Read the model definition and answer for the solid it produces. Units are mm, in the model's axes. A direction names the side the tool comes from. Coordinates: 2 decimals unless noted, no trailing zeros. Write each loop counter-clockwise with the first axis right and the second up, starting at its lowest first coordinate (ties: lowest second). Pieces come first, ordered by that corner, then holes. Notation, with made-up numbers: (2, -1) - (31, -1) arc R19 ccw to (31, 14) - close; hole circle Ø4 at (36, -5). An arc over 180 degrees is marked (long way). Use a Markdown table: item, result.
from build123d import *

# Parameters (mm, degrees)
SKETCH1_R           = 14.2875
SKETCH1_R_2         = 2.6289
BOSS_EXTRUDE1_DEPTH = 6.35


with BuildPart() as part:
    # Sketch1 → Boss-Extrude1 (new body)
    with BuildSketch(Plane(origin=(0, 0, 0), x_dir=(0, 0, -1), z_dir=(1, 0, 0))):
        with BuildLine():
            Line((-12.7, -12.7), (-88.9, -12.7))
            Line((-88.9, -12.7), (-122.826729432, 47.599537172))
            ThreePointArc((-122.826729432, 47.599537172), (-123.857351192, 50.361897296), (-123.993843813, 53.307094137))
            Line((-123.993843813, 53.307094137), (-122.611234502, 65.931609632))
            ThreePointArc((-122.611234502, 65.931609632), (-118.418396066, 72.825240039), (-110.43997975, 74.028114691))
            Line((-110.43997975, 74.028114691), (-76.479373631, 63.978142452))
            ThreePointArc((-76.479373631, 63.978142452), (-71.278861085, 61.827211414), (-66.637517322, 58.644482532))
            Line((-66.637517322, 58.644482532), (-12.7, 12.7))
            Line((-12.7, 12.7), (25.4, 12.7))
            Line((25.4, 12.7), (81.28, 12.7))
            Line((81.28, 12.7), (88.9, -12.7))
            Line((88.9, -12.7), (25.4, -12.7))
            Line((25.4, -12.7), (-12.7, -12.7))
        make_face()
        with Locations((-84.1375, 38.1)):
            Circle(SKETCH1_R, mode=Mode.SUBTRACT)
        with Locations((-12.7, 0)):
            Circle(SKETCH1_R_2, mode=Mode.SUBTRACT)
        with Locations((12.7, 0)):
            Circle(SKETCH1_R_2, mode=Mode.SUBTRACT)
        with Locations((68.58, 0)):
            Circle(SKETCH1_R_2, mode=Mode.SUBTRACT)
        with Locations((-113.142847881, 64.894652649)):
            Circle(SKETCH1_R_2, mode=Mode.SUBTRACT)
        with Locations((-114.525457191, 52.270137154)):
            Circle(SKETCH1_R_2, mode=Mode.SUBTRACT)
    extrude(amount=BOSS_EXTRUDE1_DEPTH)


solid = part.part
(1) Straight lines are drawn through the part: L1, parallel to Y at x = 4.25, z = -12.7; L2, parallel to Y at x = 5.75, z = -64; L3, parallel to Y at x = 6.25, z = 83.5. For each, find the intervals that lie inside material, in ascending order.
Report:
| item | result |
|---|---|
| L1 | y = -12.7 to -2.63, 2.63 to 12.7 |
| L2 | y = -12.7 to 12.7 |
| L3 | y = -12.7 to 23.83, 52.37 to 66.06 |
(2) A cutting plane is placed at A-A, the plane z = -68.58. Write down the section's boundary in (x, y).
Report:
| item | result |
|---|---|
| outline | (0, -12.7) - (6.35, -12.7) - (6.35, -2.63) - (0, -2.63) - close; (0, 2.63) - (6.35, 2.63) - (6.35, 12.7) - (0, 12.7) - close |
(3) Each of these flat-tipped pins is pushed along its axis until it touches: P1, Ø3, axis at x = 1.5, z = -56, coming from the +Y side; P2, Ø1.5, axis at x = 2, y = 4, coming from the -Z side (3 decimals); P3, Ø2, axis at x = 4, z = 81, coming from the +Y side. Where does it stop, or does it pass through?
Report:
| item | result |
|---|---|
| P1 | stops at y = 12.7 |
| P2 | stops at z = -84.115 |
| P3 | stops at y = 65.61 |
(4) For faces 4 (the flat face through (3, 12.7, -34)), 5 (the flat face through (3, -12.7, -1)), determine the directions among +Z, -Z, +X, -X, +Y, -Y from which every point of the face is accessible in a straight line to the end or side of a thin tool.
Report:
| item | result |
|---|---|
| face 4 | -Z, +X, -X, +Y |
| face 5 | +Z, -Z, +X, -X, -Y |
(5) A cutting plane is placed at D-D, the plane y = 0. Write down the section's boundary in (x, z).
Report:
| item | result |
|---|---|
| outline | (0, -85.09) - (6.35, -85.09) - (6.35, -71.21) - (0, -71.21) - close; (0, -65.95) - (6.35, -65.95) - (6.35, -15.33) - (0, -15.33) - close; (0, -10.07) - (6.35, -10.07) - (6.35, 10.07) - (0, 10.07) - close; (0, 15.33) - (6.35, 15.33) - (6.35, 96.05) - (0, 96.05) - close |
(6) A cutting plane is placed at C-C, the plane x = 4.5. Count the separate pieces of the cut face and the enclosed holes in it, and give its area (3 significant figures).
Report:
| item | result |
|---|---|
| separate pieces | 1 |
| enclosed holes | 6 |
| area | 7,900 mm² |
(7) A cutting plane is placed at B-B, the plane y = 38.1. Write down the section's boundary in (x, z) (3 decimals).
Report:
| item | result |
|---|---|
| outline | (0, 42.519) - (6.35, 42.519) - (6.35, 69.85) - (0, 69.85) - close; (0, 98.425) - (6.35, 98.425) - (6.35, 117.482) - (0, 117.482) - close |
(8) The mould has two halves that part along X. Classify faces 1 (the flat face through (6.35, 12, 40)), 2 (the flat face through (0, 12, 40)), 3 (the cylindrical face through (3.13, 50.32, 123.85)): pulls with the +X half, pulls with the -X half, needs draft (parallel to the pull), parting line crosses it, or undercut.
Report:
| item | result |
|---|---|
| face 1 | pulls with the +X half |
| face 2 | pulls with the -X half |
| face 3 | needs draft |
